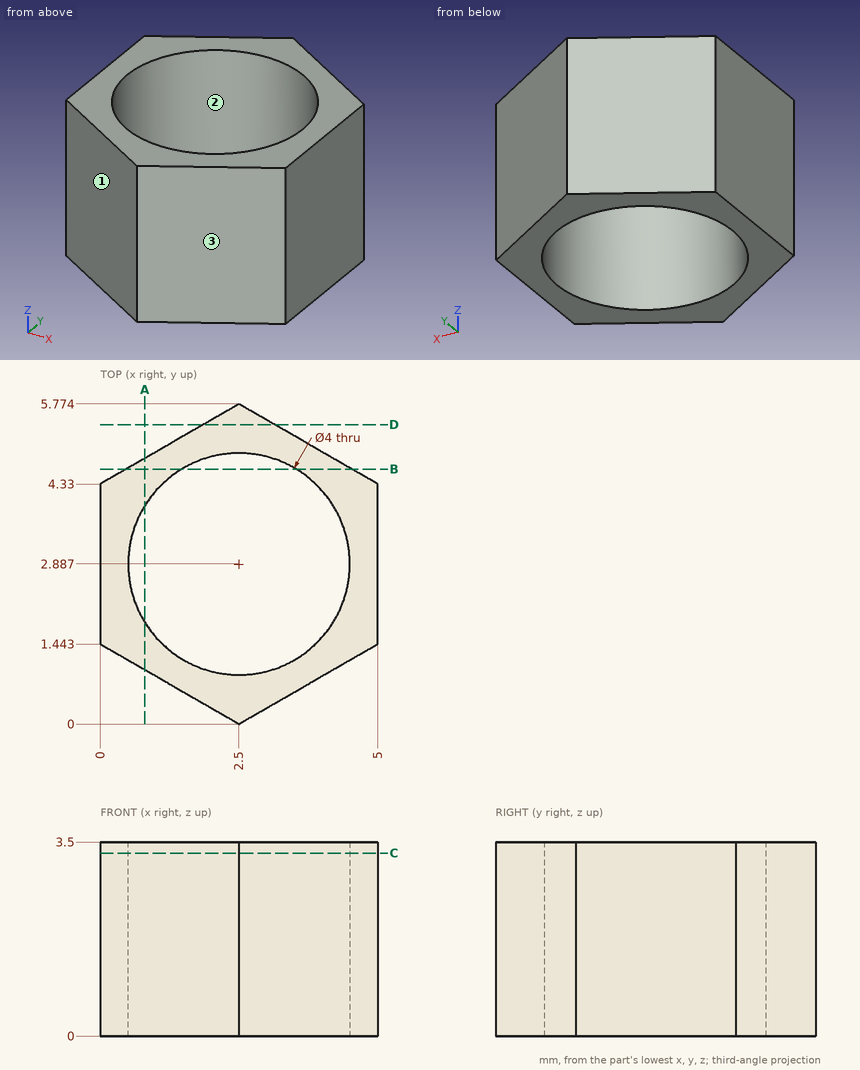
Design review of the part shown in the three views and the two pictorial views. Dimensions are in mm from the part's minimum x, y and z. Round coordinates to 2 decimals unless told otherwise and drop trailing zeros. Write each loop counter-clockwise with the first axis right and the second up, starting at its lowest first coordinate (ties: lowest second). Pieces come first, ordered by that corner, then holes.
1) Take a section at A-A on x = 0.8. Give the boundary of the cut face in (y, z).
Answer below:
outline: (0.98, 0) - (1.83, 0) - (1.83, 3.5) - (0.98, 3.5) - close; (3.94, 0) - (4.79, 0) - (4.79, 3.5) - (3.94, 3.5) - close
2) Insertion check: pin 1 Ø2.5 at (x, y) = (2.5, 2.89) entering from -Z; pin 2 Ø2 at (x, z) = (3, 1.5) entering from -Y; pin 3 Ø3 at (x, y) = (3, 4) entering from -Z. Each pin has a flat end and moves straight along its axis. Give the tip position at first contact, or say it passes through.
Answer below:
pin 1: passes through
pin 2: stops at y = 0
pin 3: stops at z = 0
3) Take a section at C-C on z = 3.3. Give the boundary of the cut face in (x, y).
Answer below:
outline: (0, 1.44) - (2.5, 0) - (5, 1.44) - (5, 4.33) - (2.5, 5.77) - (0, 4.33) - close; hole circle Ø4 at (2.5, 2.89)
4) For line 1 along X through (y, z) = (1.65, 3.15); line 2 along X through (y, z) = (3, 0.45); line 3 along Y through (x, z) = (3.7, 0.5) (1 decimal), list the stretches that pass through material, from the lowest coordinate up.
Answer below:
line 1: x = 0 to 0.93, 4.07 to 5
line 2: x = 0 to 0.5, 4.5 to 5
line 3: y = 0.7 to 1.3, 4.5 to 5.1
5) Take a section at D-D on y = 5.4. Give the boundary of the cut face in (x, z).
Answer below:
outline: (1.85, 0) - (3.15, 0) - (3.15, 3.5) - (1.85, 3.5) - close
6) Mouldability with a two-part tool opening along X and no side actions: class the marked faces 1, 2 and 3 as +X half, -X half, draft (parallel to the pull), parting line (faces both ways), or undercut.
Answer below:
face 1: -X half
face 2: undercut
face 3: +X half
7) Take a section at B-B on y = 4.6. Give the boundary of the cut face in (x, z).
Answer below:
outline: (0.47, 0) - (1.47, 0) - (1.47, 3.5) - (0.47, 3.5) - close; (3.53, 0) - (4.53, 0) - (4.53, 3.5) - (3.53, 3.5) - close
